For this review, take the finished solid that the model builds, in its own axes (mm). A direction names the side the tool comes from. Give positions to 0.01 mm unless a question says otherwise; leave off trailing zeros. Loops run counter-clockwise (first coordinate to the right, second up) from the corner with the lowest first, then second, coordinate; pieces in that order, holes last. Notation, with made-up numbers: (79, -35) - (95, -35) arc R19 ccw to (95, -2) - close; hole circle Ø7 at (-12.5, 85). An arc over 180 degrees is marked (long way). Use CSV: the item, a comma, the result in double quotes. Start each with the question number.
1. Take a section at C-C on z = 10.5. Give the boundary of the cut face in (x, y).
2. Wall thickness on line 1 (X direction, y = -3.25, z = 126); line 2 (Y direction, x = 81.5, z = 64); line 3 (Z direction, x = 108.5, y = -5.5): over which ranges is each line inside the solid? List them lowest first.
3. For pin 1 (2 mm diameter, centred on x = 111, z = 99, fed in from -Y); pin 2 (4 mm diameter, centred on x = 77, y = -8, fed in from -Z), all flat-tipped, find the tip position at first contact; note any pin that passes through.
4. Take a section at B-B on y = -2.5. Give the boundary of the cut face in (x, z), plus the area to 3 significant figures.
5. Mouldability with a two-part tool opening along X and no side actions: class faces 1 (the flat face through (0, -4, 69)), 2 (the flat face through (61, 1, 69)), 3 (the flat face through (123, -4, 69)) as pulls with the +X half, pulls with the -X half, needs draft (parallel to the pull), parting line crosses it, or undercut.
6. Take a section at A-A on x = 14.5. Give the boundary of the cut face in (y, z).
7. For faces 4 (the flat face through (62.3, 0.5, 0)), 5 (the flat face through (63, -4, 139)), list the 3-axis set-ups (+Z, -Z, +X, -X, +Y, -Y) from which the entire face can be reached by the end or side of a thin tool; tool diameter is ignored.
```python
from build123d import *

# Parameters (mm, degrees)
SZKIC1_W                    = 124
SZKIC1_H                    = 140
DODANIE_WYCI_GNI_CIE1_DEPTH = 1
DODANIE_WYCI_GNI_CIE2_DEPTH = 10


with BuildPart() as part:
    # Szkic1 → Dodanie-wyciągnięcie1 (new body)
    with BuildSketch(Plane(origin=(0, 0, 0), x_dir=(1, 0, 0), z_dir=(0, 1, 0))):
        with Locations((62, -70)):
            Rectangle(SZKIC1_W, SZKIC1_H)
    extrude(amount=DODANIE_WYCI_GNI_CIE1_DEPTH)

    # Szkic3 → Dodanie-wyciągnięcie2 (add)
    with BuildSketch(Plane(origin=(0, 1, 0), x_dir=(1, 0, 0), z_dir=(0, 1, 0))):
        Polygon((0, 0), (0, -140), (124, -140), (124, 0), (123, 0), (123, -139), (1, -139), (1, 0), align=None)
    extrude(amount=-DODANIE_WYCI_GNI_CIE2_DEPTH)


solid = part.part
```
Check result:
1,outline,"(0, -9) - (1, -9) - (1, 0) - (123, 0) - (123, -9) - (124, -9) - (124, 1) - (0, 1) - close"
2,line 1,"x = 0 to 1, 123 to 124"
2,line 2,"y = 0 to 1"
2,line 3,"z = 139 to 140"
3,pin 1,"stops at y = 0"
3,pin 2,"stops at z = 139"
4,outline,"(0, 0) - (1, 0) - (1, 139) - (123, 139) - (123, 0) - (124, 0) - (124, 140) - (0, 140) - close"
4,area,"402 mm²"
5,face 1,"pulls with the -X half"
5,face 2,"needs draft"
5,face 3,"undercut"
6,outline,"(-9, 139) - (0, 139) - (0, 0) - (1, 0) - (1, 140) - (-9, 140) - close"
7,face 4,"-Z, +X, -X, +Y, -Y"
7,face 5,"-Z, -Y"
